Here's how the part is built. I have some questions about the finished solid (model axes, mm). Face numbers are marked on the shaded views. Round coordinates to 2 decimals unless told otherwise and drop trailing zeros. Write each loop counter-clockwise with the first axis right and the second up, starting at its lowest first coordinate (ties: lowest second). Pieces come first, ordered by that corner, then holes. Notation, with made-up numbers: M 57,-34.75 L 90,-34.75 A12 ccw 90,-21.75 Z; hole C 35.5,-12 d3. An arc over 180 degrees is marked long. Use one line per item in the form item = value. Start each with the question number.
Q1. I need wall thicknesses on line 1 along Z through (x, y) = (-0.5, 57); line 2 along Y through (x, z) = (-86, -33). Which ranges of each line are inside material? Lowest first, please. Write a range as from..to.
Q2. I'm going to push flat-ended pins straight in: pin 1 Ø12 at (x, y) = (-75.5, 79) entering from -Z; pin 2 Ø1 at (y, z) = (40.5, 60) entering from +X; pin 3 Ø1.5 at (y, z) = (120.5, 63) entering from +X; pin 4 Ø4 at (x, z) = (-37.52, -68.49) entering from -Y. Where does each tip first touch, or does it pass through?
Q3. I want a section at D-D on z = 53. List the corners of the cut face in (x, y) for me, and give its area (3 significant figures).
Q4. We'd pull the mould along X, two halves only. Please class the marked faces 1, 2 and 3: +X half, -X half, draft (parallel to the pull), parting line (faces both ways), or undercut.
Q5. I want a section at A-A on x = 0. List the corners of the cut face in (y, z) for me, and give its area (3 significant figures).
Q6. I want a section at B-B on y = 102.5. List the corners of the cut face in (x, z) for me.
Q7. I want a section at C-C on z = 95. List the corners of the cut face in (x, y) for me.
```python
from build123d import *

# Parameters (mm, degrees)
SKETCH1_W           = 250
SKETCH1_H           = 250
BOSS_EXTRUDE1_DEPTH = 5
SKETCH8_R           = 7.5
BOSS_EXTRUDE3_DEPTH = 5
FILLET6_R           = 2
FILLET7_R           = 0.5
SKETCH11_R          = 2.5
CUT_EXTRUDE4_DEPTH  = 10
SKETCH12_OUTSIDE_W  = 322.738
SKETCH12_OUTSIDE_H  = 322.738
SKETCH12_OUTSIDE_R  = 125
CUT_EXTRUDE5_DEPTH  = 10
SKETCH13_R          = 140
SKETCH13_R_2        = 125
BOSS_EXTRUDE4_DEPTH = 175


with BuildPart() as part:
    # Sketch1 → Boss-Extrude1 (new body)
    with BuildSketch(Plane(origin=(0, 0, 0), x_dir=(1, 0, 0), z_dir=(0, 1, 0))):
        Rectangle(SKETCH1_W, SKETCH1_H)
    extrude(amount=BOSS_EXTRUDE1_DEPTH)

    # Sketch8 → Boss-Extrude3 (add)
    with BuildSketch(Plane(origin=(0, 5, 0), x_dir=(1, 0, 0), z_dir=(0, 1, 0))):
        with Locations(Location((99.778960279, -1.147118049, 0), (0, 0, 90))):
            Circle(SKETCH8_R)
        with Locations(Location((0, -95, 0), (0, 0, 90))):
            Circle(SKETCH8_R)
    extrude(amount=BOSS_EXTRUDE3_DEPTH)

    # Sketch9 → Cut-Revolve3 (revolve, cut)
    with BuildSketch(Plane(origin=(0, 0, 0), x_dir=(0, 0, -1), z_dir=(1, 0, 0))):
        with BuildLine():
            Line((-95, 15), (-95, 5))
            ThreePointArc((-95, 5), (-100, 10), (-95, 15))
        make_face()
    revolve(axis=Axis((0, 10, 95), (0, -1, 0)), mode=Mode.SUBTRACT)

    # Sketch10 → Cut-Revolve4 (revolve, cut)
    with BuildSketch(Plane.XY.offset(1.05)):
        with BuildLine():
            Line((99.778960279, 15), (99.778960279, 5))
            ThreePointArc((99.778960279, 5), (94.778960279, 10), (99.778960279, 15))
        make_face()
    revolve(axis=Axis((99.778960279, 15, 1.05), (0, -1, 0)), mode=Mode.SUBTRACT)

    # Fillet6
    fillet6_edges = [part.edges().sort_by_distance(p)[0] for p in [
        (99.778960279, 5, 8.647118049),
        (0, 5, 102.5),
    ]]
    fillet(fillet6_edges, radius=FILLET6_R)

    # Fillet7
    fillet7_edges = [part.edges().sort_by_distance(p)[0] for p in [
        (99.778960279, 10, 8.647118049),
        (0, 10, 102.5),
    ]]
    fillet(fillet7_edges, radius=FILLET7_R)

    # Sketch11 → Cut-Extrude4 (cut)
    with BuildSketch(Plane(origin=(0, 5, 0), x_dir=(1, 0, 0), z_dir=(0, 1, 0))):
        with Locations(Location((-19.240698593, 30.202545091, 0), (0, 0, 270))):
            Circle(SKETCH11_R)
        with Locations(Location((-37.517445985, 68.490408766, 0), (0, 0, 270))):
            Circle(SKETCH11_R)
        with Locations(Location((-47.523004126, 40.208103233, 0), (0, 0, 270))):
            Circle(SKETCH11_R)
        with Locations(Location((-9.235140451, 58.484850625, 0), (0, 0, 270))):
            Circle(SKETCH11_R)
    extrude(amount=-CUT_EXTRUDE4_DEPTH, mode=Mode.SUBTRACT)

    # Sketch12 outside → Cut-Extrude5 (cut)
    with BuildSketch(Plane(origin=(0, 0, 0), x_dir=(-1, 0, 0), z_dir=(0, -1, 0))):
        Rectangle(SKETCH12_OUTSIDE_W, SKETCH12_OUTSIDE_H)
        with Locations(Location((0, 0, 0), (0, 0, 90))):
            Circle(SKETCH12_OUTSIDE_R, mode=Mode.SUBTRACT)
    extrude(amount=-CUT_EXTRUDE5_DEPTH, mode=Mode.SUBTRACT)

    # Sketch13 → Boss-Extrude4 (add)
    with BuildSketch(Plane.XZ):
        with Locations(Location((0, 0, 0), (0, 0, 270))):
            Circle(SKETCH13_R)
        with Locations(Location((0, 0, 0), (0, 0, 270))):
            Circle(SKETCH13_R_2, mode=Mode.SUBTRACT)
    extrude(amount=-BOSS_EXTRUDE4_DEPTH)


solid = part.part
```
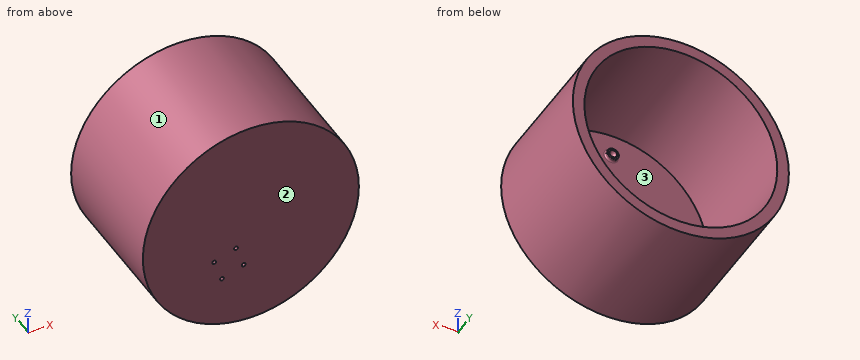
Reported:
q1.line_1 = -140..-125, 125..140
q1.line_2 = 0..5
q2.pin_1 = -121.53
q2.pin_2 = 126.73
q2.pin_3 = 125.4
q2.pin_4 = through
q3.outline = M -129.58,0 L 129.58,0 L 129.58,175 L 113.21,175 L 113.21,5 L -113.21,5 L -113.21,175 L -129.58,175 Z
q3.area = 6,860 mm^2
q4.face_1 = parting line
q4.face_2 = draft
q4.face_3 = undercut
q5.outline = M 0,-140 L 175,-140 L 175,-125 L 5,-125 L 5,85.5 A2 cw 7,87.5 L 9.5,87.5 A0.5 ccw 10,88 L 10,90 A5 cw 10,100 L 10,102 A0.5 ccw 9.5,102.5 L 7,102.5 A2 cw 5,104.5 L 5,125 L 175,125 L 175,140 L 0,140 Z
q5.area = 6,540 mm^2
q6.outline = C 0,0 d280; hole C 0,0 d250
q7.outline = M -102.83,0 L 102.83,0 L 102.83,175 L 81.24,175 L 81.24,5 L 9.5,5 A2 cw 7.5,7 L 7.5,9.5 A0.5 ccw 7,10 L 5,10 A5 cw -5,10 L -7,10 A0.5 ccw -7.5,9.5 L -7.5,7 A2 cw -9.5,5 L -81.24,5 L -81.24,175 L -102.83,175 Z
